Can you work these out from the drawing? Everything is in mm from the part's minimum corner. Round coordinates to 2 decimals unless told otherwise and drop trailing zeros. Write each loop counter-clockwise with the first axis right and the second up, starting at its lowest first coordinate (ties: lowest second). Pieces come first, ordered by that corner, then holes. Notation, with made-up numbers: (56.5, 40) -> (108.5, 40) arc R14 ccw to (108.5, 64) -> close; hole circle Ø6 at (87.5, 40). An arc over 180 degrees is marked (long way). Write item = value, one per line. Start each with the question number.
1) Imagine slicing it at C-C, the plane x = 80. Please give me the cut outline in (y, z), then the cut area to 3 significant figures.
2) Imagine slicing it at B-B, the plane z = 6.25. Please give me the cut outline in (x, y), then the cut area to 4 significant figures.
3) Imagine slicing it at A-A, the plane y = 44.45. Please give me the cut outline in (x, z), then the cut area to 3 significant figures.
4) If I drill on line 1 (Y direction, x = 385.5, z = 17.5); line 2 (Y direction, x = 86, z = 4), over which ranges is the centre line in solid material (lowest first)?
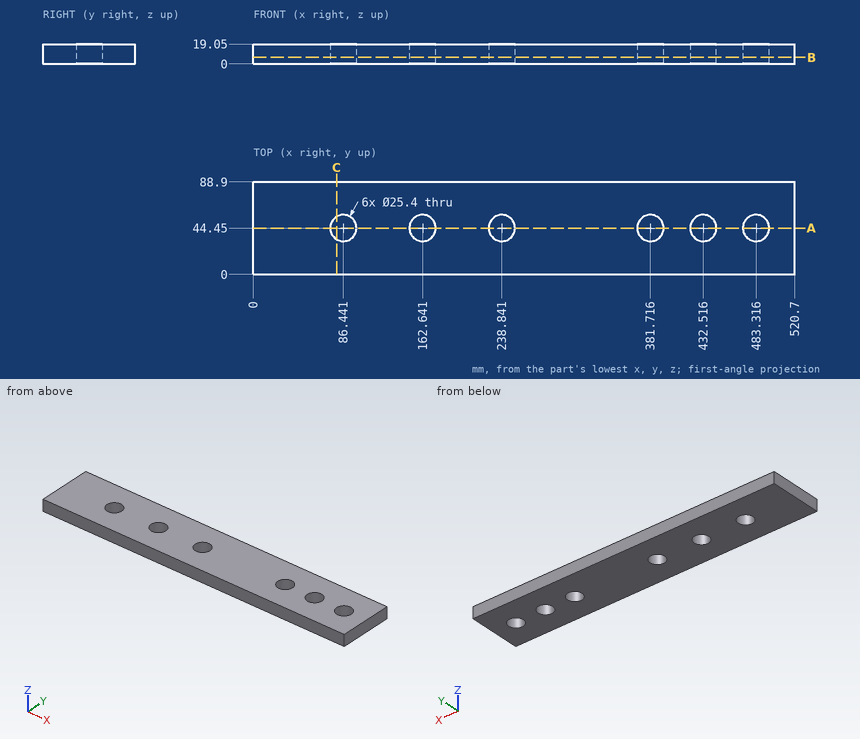
Reported:
q1.outline = (0, 0) -> (33.5, 0) -> (33.5, 19.05) -> (0, 19.05) -> close; (55.4, 0) -> (88.9, 0) -> (88.9, 19.05) -> (55.4, 19.05) -> close
q1.area = 1,280 mm²
q2.outline = (0, 0) -> (520.7, 0) -> (520.7, 88.9) -> (0, 88.9) -> close; hole circle Ø25.4 at (86.44, 44.45); hole circle Ø25.4 at (162.64, 44.45); hole circle Ø25.4 at (238.84, 44.45); hole circle Ø25.4 at (381.72, 44.45); hole circle Ø25.4 at (432.52, 44.45); hole circle Ø25.4 at (483.32, 44.45)
q2.area = 43,250 mm²
q3.outline = (0, 0) -> (73.74, 0) -> (73.74, 19.05) -> (0, 19.05) -> close; (99.14, 0) -> (149.94, 0) -> (149.94, 19.05) -> (99.14, 19.05) -> close; (175.34, 0) -> (226.14, 0) -> (226.14, 19.05) -> (175.34, 19.05) -> close; (251.54, 0) -> (369.02, 0) -> (369.02, 19.05) -> (251.54, 19.05) -> close; (394.42, 0) -> (419.82, 0) -> (419.82, 19.05) -> (394.42, 19.05) -> close; (445.22, 0) -> (470.62, 0) -> (470.62, 19.05) -> (445.22, 19.05) -> close; (496.02, 0) -> (520.7, 0) -> (520.7, 19.05) -> (496.02, 19.05) -> close
q3.area = 7,020 mm²
q4.line_1 = 0 to 32.33, 56.57 to 88.9
q4.line_2 = 0 to 31.76, 57.14 to 88.9
